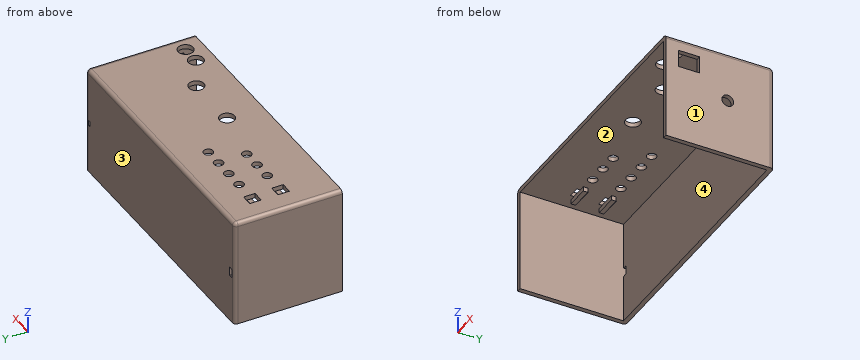
from build123d import *

# Parameters (mm, degrees)
BOSS_EXTRUDE1_DEPTH = 55
SKETCH3_W           = 9.2
SKETCH3_H           = 11.2
CUT_EXTRUDE1_DEPTH  = 2.4
SKETCH4_R           = 4
CUT_EXTRUDE2_DEPTH  = 2.4
SKETCH5_R           = 2.5
CUT_EXTRUDE3_DEPTH  = 2.4
SKETCH7_R           = 4
CUT_EXTRUDE4_DEPTH  = 2.4
SKETCH8_W           = 6.1
SKETCH8_H           = 6.1
CUT_EXTRUDE5_DEPTH  = 2.4
SKETCH9_W           = 12
SKETCH9_H           = 2.4
BOSS_EXTRUDE3_DEPTH = 2.4
SKETCH10_R          = 4
CUT_EXTRUDE6_DEPTH  = 2.4
BOSS_EXTRUDE4_DEPTH = 2.4
SKETCH12_W          = 1.5
SKETCH12_H          = 3
SKETCH12_W_2        = 2.4
SKETCH12_H_2        = 4.8
CUT_EXTRUDE7_DEPTH  = 2.4
SKETCH13_R          = 3.125
CUT_EXTRUDE8_DEPTH  = 2.4
FILLET1_R           = 2


with BuildPart() as part:
    # Sketch2 → Boss-Extrude1 (new body)
    with BuildSketch(Plane(origin=(0, 0, 0), x_dir=(1, 0, 0), z_dir=(0, 1, 0))):
        with BuildLine():
            Line((-70, 55), (-70, 0))
            Line((-70, 0), (70, 0))
            Line((70, 0), (70, 55))
            Line((70, 55), (72.4, 55))
            Line((72.4, 55), (72.4, -0.4))
            ThreePointArc((72.4, -0.4), (71.814213562, -1.814213562), (70.4, -2.4))
            Line((70.4, -2.4), (-70.4, -2.4))
            ThreePointArc((-70.4, -2.4), (-71.814213562, -1.814213562), (-72.4, -0.4))
            Line((-72.4, -0.4), (-72.4, 55))
            Line((-72.4, 55), (-70, 55))
        make_face()
    extrude(amount=BOSS_EXTRUDE1_DEPTH)

    # Sketch3 → Cut-Extrude1 (cut)
    with BuildSketch(Plane(origin=(72.4, 0, 0), x_dir=(0, 0, -1), z_dir=(1, 0, 0))):
        with Locations((8.964963507, 12.3)):
            Rectangle(SKETCH3_W, SKETCH3_H)
    extrude(amount=-CUT_EXTRUDE1_DEPTH, mode=Mode.SUBTRACT)

    # Sketch4 → Cut-Extrude2 (cut)
    with BuildSketch(Plane.XY.offset(2.4)):
        with Locations((53.50014494, 9.325)):
            Circle(SKETCH4_R)
        with Locations((35.20014494, 19.025)):
            Circle(SKETCH4_R)
    extrude(amount=-CUT_EXTRUDE2_DEPTH, mode=Mode.SUBTRACT)

    # Sketch5 → Cut-Extrude3 (cut)
    with BuildSketch(Plane.XY.offset(2.4)):
        with Locations((-45, 25)):
            Circle(SKETCH5_R)
        with Locations((-35, 25)):
            Circle(SKETCH5_R)
        with Locations((-25, 25)):
            Circle(SKETCH5_R)
        with Locations((-35, 40)):
            Circle(SKETCH5_R)
        with Locations((-25, 40)):
            Circle(SKETCH5_R)
        with Locations((-15, 40)):
            Circle(SKETCH5_R)
        with Locations((-45, 40)):
            Circle(SKETCH5_R)
    extrude(amount=-CUT_EXTRUDE3_DEPTH, mode=Mode.SUBTRACT)

    # Sketch7 → Cut-Extrude4 (cut)
    with BuildSketch(Plane.XY.offset(2.4)):
        with Locations((5.20014494, 19.025)):
            Circle(SKETCH7_R)
    extrude(amount=-CUT_EXTRUDE4_DEPTH, mode=Mode.SUBTRACT)

    # Sketch8 → Cut-Extrude5 (cut)
    with BuildSketch(Plane.XY.offset(2.4)):
        with Locations((-58.05, 25)):
            Rectangle(SKETCH8_W, SKETCH8_H)
        with Locations((-58.05, 40)):
            Rectangle(SKETCH8_W, SKETCH8_H)
    extrude(amount=-CUT_EXTRUDE5_DEPTH, mode=Mode.SUBTRACT)

    # Sketch9 → Boss-Extrude3 (add)
    with BuildSketch(Plane(origin=(0, 0, 0), x_dir=(-1, 0, 0), z_dir=(0, 0, -1))):
        with Locations((58.05, 25)):
            Rectangle(SKETCH9_W, SKETCH9_H)
        with Locations((58.05, 40)):
            Rectangle(SKETCH9_W, SKETCH9_H)
    extrude(amount=BOSS_EXTRUDE3_DEPTH)

    # Sketch10 → Cut-Extrude6 (cut)
    with BuildSketch(Plane.XY.offset(2.4)):
        with Locations((63.50014494, 9.325)):
            Circle(SKETCH10_R)
    extrude(amount=-CUT_EXTRUDE6_DEPTH, mode=Mode.SUBTRACT)

    # Sketch11 → Boss-Extrude4 (add)
    with BuildSketch(Plane(origin=(0, 55, 0), x_dir=(1, 0, 0), z_dir=(0, 1, 0))):
        with BuildLine():
            Line((-72.4, 55), (72.4, 55))
            Line((72.4, 55), (72.4, -0.4))
            ThreePointArc((72.4, -0.4), (71.814213562, -1.814213562), (70.4, -2.4))
            Line((70.4, -2.4), (-70.4, -2.4))
            ThreePointArc((-70.4, -2.4), (-71.814213562, -1.814213562), (-72.4, -0.4))
            Line((-72.4, -0.4), (-72.4, 55))
        make_face()
    extrude(amount=BOSS_EXTRUDE4_DEPTH)

    # Sketch12 → Cut-Extrude7 (cut)
    with BuildSketch(Plane(origin=(0, 57.4, 0), x_dir=(1, 0, 0), z_dir=(0, 1, 0))):
        with Locations((69.25, 27.3)):
            Rectangle(SKETCH12_W, SKETCH12_H)
        with Locations((-68.8, 27.3)):
            Rectangle(SKETCH12_W_2, SKETCH12_H_2)
    extrude(amount=-CUT_EXTRUDE7_DEPTH, mode=Mode.SUBTRACT)

    # Sketch13 → Cut-Extrude8 (cut)
    with BuildSketch(Plane(origin=(72.4, 0, 0), x_dir=(0, 0, -1), z_dir=(1, 0, 0))):
        with Locations((24.364963507, 32.9)):
            Circle(SKETCH13_R)
    extrude(amount=-CUT_EXTRUDE8_DEPTH, mode=Mode.SUBTRACT)

    # Fillet1
    fillet1_edges = [part.edges().sort_by_distance(p)[0] for p in [
        (-72.4, 57.4, -27.3),
        (-71.814213562, 57.4, 1.814213562),
        (0, 57.4, 2.4),
        (71.814213562, 57.4, 1.814213562),
        (72.4, 57.4, -27.3),
    ]]
    fillet(fillet1_edges, radius=FILLET1_R)


solid = part.part
The model under review builds one solid part; all positions refer to its coordinate system, in mm. Face numbers are marked on the shaded views. Round coordinates to 2 decimals unless told otherwise and drop trailing zeros. Loops run counter-clockwise (first coordinate to the right, second up) from the corner with the lowest first, then second, coordinate; pieces in that order, holes last. Notation, with made-up numbers: (29, -18) -> (74, -18) arc R4 cw to (74, -13) -> close; hole circle Ø7 at (48, 51). An arc over 180 degrees is marked (long way). Answer as CSV lines item,"result".
1) To check wall thickness, follow line 1 along Y through (x, z) = (-54.5, -2); line 2 along X through (y, z) = (52, -21); line 3 along Y through (x, z) = (35.5, -25.5). State the ranges of each line that lie inside material, in increasing order. Write a range as from..to.
Geometry results:
line 1,"y = 23.8..26.2, 38.8..41.2, 55..57.4"
line 2,"x = -72.4..-70, 70..72.4"
line 3,"y = 55..57.4"
2) Add section B-B on y = 32.9. Write out the cut boundary in (x, z), plus the area to 3 significant figures.
Geometry results:
outline,"(-72.4, -55) -> (-70, -55) -> (-70, 0) -> (70, 0) -> (70, -21.24) -> (72.4, -21.24) -> (72.4, 0.4) arc R2 ccw to (70.4, 2.4) -> (-70.4, 2.4) arc R2 ccw to (-72.4, 0.4) -> close; (70, -55) -> (72.4, -55) -> (72.4, -27.49) -> (70, -27.49) -> close"
area,"595 mm²"
3) Draft analysis for pull direction X (two halves, no side actions). For the marked faces 1, 2, 3 and 4, state which applies: pulls with the +X half, pulls with the -X half, needs draft (parallel to the pull), parting line crosses it, or undercut.
Geometry results:
face 1,"pulls with the +X half"
face 2,"undercut"
face 3,"needs draft"
face 4,"undercut"
4) Add section D-D on z = -36. Write out the cut boundary in (x, y).
Geometry results:
outline,"(-72.4, 0) -> (-70, 0) -> (-70, 55) -> (70, 55) -> (70, 0) -> (72.4, 0) -> (72.4, 55.4) arc R2 ccw to (70.4, 57.4) -> (-70.4, 57.4) arc R2 ccw to (-72.4, 55.4) -> close"
5) Add section A-A on x = -45. Write out the cut boundary in (y, z), plus the area to 3 significant figures.
Geometry results:
outline,"(0, 0) -> (22.5, 0) -> (22.5, 2.4) -> (0, 2.4) -> close; (27.5, 0) -> (37.5, 0) -> (37.5, 2.4) -> (27.5, 2.4) -> close; (42.5, 0) -> (55, 0) -> (55, -55) -> (57.4, -55) -> (57.4, 0.4) arc R2 ccw to (55.4, 2.4) -> (42.5, 2.4) -> close"
area,"245 mm²"
6) Add section C-C on x = 54. Write out the cut boundary in (y, z), plus the area to 3 significant figures.
Geometry results:
outline,"(0, 0) -> (5.36, 0) -> (5.36, 2.4) -> (0, 2.4) -> close; (13.29, 0) -> (55, 0) -> (55, -55) -> (57.4, -55) -> (57.4, 0.4) arc R2 ccw to (55.4, 2.4) -> (13.29, 2.4) -> close"
area,"250 mm²"
7) For P1, Ø2, axis at x = 28, y = 46, coming from the -Z side; P2, Ø1.2, axis at x = -57.5, y = 25, coming from the +Z side; P3, Ø0.7, axis at y = 24.5, z = 1.5, coming from the +X side, all flat-tipped, find the tip position at first contact; note any pin that passes through.
Geometry results:
P1,"stops at z = 0"
P2,"stops at z = 0"
P3,"stops at x = 72.25"
